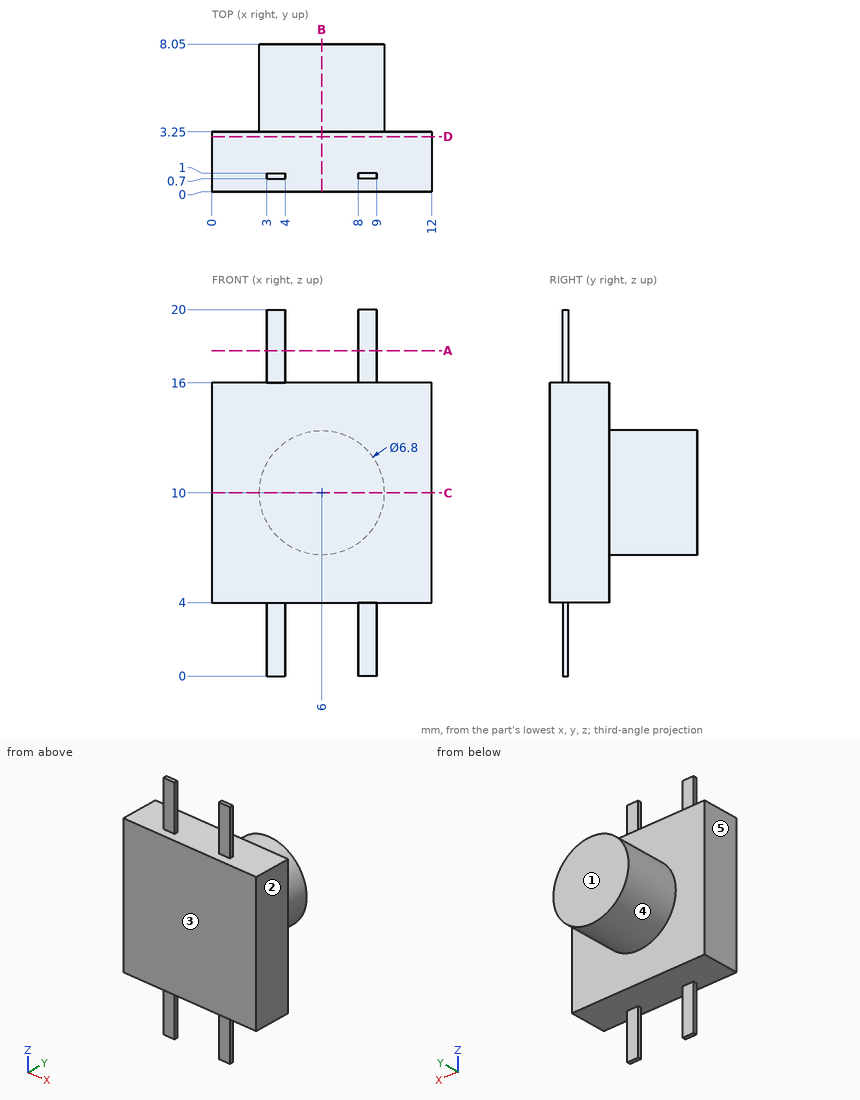
Job drawing, mm, ordinate dimensions from the low corner. One solid piece. A direction names the side the tool comes from. Give positions to 0.01 mm unless a question says otherwise; leave off trailing zeros. Loops run counter-clockwise (first coordinate to the right, second up) from the corner with the lowest first, then second, coordinate; pieces in that order, holes last. Notation, with made-up numbers: (85, -9.75) -> (118, -9.75) arc R11 cw to (118, 6.25) -> close; hole circle Ø5 at (14, -1). An arc over 180 degrees is marked (long way). Write each question's results on one line, items separated by ' | '. Start each with the question number.
Q1. Band-saw the part on D-D on y = 3. List the corners of the cut face in (x, z), plus the area to 3 significant figures.
Q2. Which spindle directions (+Z, -Z, +X, -X, +Y, -Y) get a long thin tool onto all of the face, cutting with end or side? Do the marked faces 4 and 5. Say none if no direction does.
Q3. Band-saw the part on C-C on z = 10. List the corners of the cut face in (x, y).
Q4. Pull direction Y, two halves, no side cores. Call the marked faces 1, 2 and 3: +Y half, -Y half, draft (parallel to the pull), parting line (faces both ways), or undercut.
Q5. Band-saw the part on A-A on z = 17.75. List the corners of the cut face in (x, y), plus the area to 3 significant figures.
Q6. Band-saw the part on B-B on x = 6. List the corners of the cut face in (y, z).
Q7. Wall check: L1, parallel to Y at x = 1.5, z = 6.5; L2, parallel to Z at x = 6.75, y = 3; L3, parallel to Z at x = 5, y = 4. Give the ranges that are in metal, low to high.
Q8. Pin check, flat tips, straight feed: P1, Ø1.1, axis at x = 8.5, z = 2, coming from the -Y side; P2, Ø4, axis at y = 6.5, z = 10.5, coming from the +X side; P3, Ø0.5, axis at x = 8.5, z = 2.5, coming from the +Y side. Stop position of each tip, or through.
Results are:
1) outline: (0, 4) -> (12, 4) -> (12, 16) -> (0, 16) -> close | area: 144 mm²
2) face 4: +Y | face 5: +Z, -Z, -X, +Y, -Y
3) outline: (0, 0) -> (12, 0) -> (12, 3.25) -> (9.4, 3.25) -> (9.4, 8.05) -> (2.6, 8.05) -> (2.6, 3.25) -> (0, 3.25) -> close
4) face 1: +Y half | face 2: draft | face 3: -Y half
5) outline: (3, 0.7) -> (4, 0.7) -> (4, 1) -> (3, 1) -> close; (8, 0.7) -> (9, 0.7) -> (9, 1) -> (8, 1) -> close | area: 0.600 mm²
6) outline: (0, 4) -> (3.25, 4) -> (3.25, 6.6) -> (8.05, 6.6) -> (8.05, 13.4) -> (3.25, 13.4) -> (3.25, 16) -> (0, 16) -> close
7) L1: y = 0 to 3.25 | L2: z = 4 to 16 | L3: z = 6.75 to 13.25
8) P1: stops at y = 0.7 | P2: stops at x = 9.4 | P3: stops at y = 1
